from build123d import *

# Parameters (mm, degrees)
F1_DEPTH = 5
F2_T     = -2.5
F3_R     = 7
F4_R     = 7
F5_R     = 10
F6_R     = 10
F7_R     = 7
F8_R     = 7
F9_R     = 4.99999


# Not quite as in the source:
# - a fillet or chamfer is up to 0.001 mm smaller than in the source, because OpenCascade refuses the exact size


with BuildPart() as f1:
    # F0 (on Top) → F1 (new body)
    with BuildSketch(Plane.XY):
        Polygon((25, 55), (-25, 55), (-40, -5), (-25, -55), (25, -55), (40, -5), align=None)
    extrude(amount=F1_DEPTH)

    # F2
    f2_openings = [f1.faces().sort_by_distance(p)[0] for p in [
        (0, -0.384615, 5),
    ]]
    offset(amount=F2_T, openings=f2_openings)

    # F3
    f3_edges = [f1.edges().sort_by_distance(p)[0] for p in [
        (25, 55, 2.5),
    ]]
    fillet(f3_edges, radius=F3_R)

    # F4
    f4_edges = [f1.edges().sort_by_distance(p)[0] for p in [
        (-25, 55, 2.5),
    ]]
    fillet(f4_edges, radius=F4_R)

    # F5
    f5_edges = [f1.edges().sort_by_distance(p)[0] for p in [
        (-40, -5, 2.5),
    ]]
    fillet(f5_edges, radius=F5_R)

    # F6
    f6_edges = [f1.edges().sort_by_distance(p)[0] for p in [
        (40, -5, 2.5),
    ]]
    fillet(f6_edges, radius=F6_R)

    # F7
    f7_edges = [f1.edges().sort_by_distance(p)[0] for p in [
        (-25, -55, 2.5),
    ]]
    fillet(f7_edges, radius=F7_R)

    # F8
    f8_edges = [f1.edges().sort_by_distance(p)[0] for p in [
        (25, -55, 2.5),
    ]]
    fillet(f8_edges, radius=F8_R)

    # F9 (radius 5 in the source; OpenCascade refuses exactly that, so slightly less here)
    f9_edges = [f1.edges().sort_by_distance(p)[0] for p in [
        (32.853411, -28.821964, 0),
    ]]
    fillet(f9_edges, radius=F9_R)


solid = f1.part
The model under review builds one solid part; all positions refer to its coordinate system, in mm. A direction names the side the tool comes from. Round coordinates to 2 decimals unless told otherwise and drop trailing zeros. Return JSON: item names as keys, results as strings.
1. The part is to be moulded in two halves that separate along Y. For faces 3 (the face through (-31.324, -28.687, 1.426)), 4 (the face through (0, 52.5, 4)), 5 (the face through (-31.462, 22.953, 1.426)), say which applies: +Y half, -Y half, draft (parallel to the pull), parting line (faces both ways), or undercut.
Answer block:
{"face 3": "-Y half", "face 4": "undercut", "face 5": "+Y half"}
2. For faces 1 (the face through (30.33, 23.38, 3.73)), 2 (the face through (0, -53, 1)), list the 3-axis set-ups (+Z, -Z, +X, -X, +Y, -Y) from which the entire face can be reached by the end or side of a thin tool; tool diameter is ignored.
Answer block:
{"face 1": "+Z", "face 2": "-Z, +X, -X, -Y"}
3. Insertion check: P1, Ø1, axis at y = -21.5, z = 0.5, coming from the +X side; P2, Ø1.5, axis at x = -25, z = 2.5, coming from the +Y side; P3, Ø1, axis at x = 1, z = 1.5, coming from the +Y side. Each pin has a flat end and moves straight along its axis. Give the tip position at first contact, or say it passes through.
Answer block:
{"P1": "stops at x = 32.98", "P2": "stops at y = 52.4", "P3": "stops at y = 54"}
4. For L1, parallel to Z at x = -11, y = 2; L2, parallel to Y at x = 20.5, z = 3.25; L3, parallel to X at y = 43, z = 3.3, list the stretches that pass through material, from the lowest coordinate up. Write a range as [from, to].
Answer block:
{"L1": "z = [0, 2.5]", "L2": "y = [-54.65, -52.5], [52.5, 54.61]", "L3": "x = [-27.69, -25.42], [25.42, 27.69]"}
